Geometry: final body of the model. Coordinates: model frame, mm. A direction names the side the tool comes from. Give positions to 0.01 mm unless a question says otherwise; leave off trailing zeros. Write each loop counter-clockwise with the first axis right and the second up, starting at its lowest first coordinate (ties: lowest second). Pieces come first, ordered by that corner, then holes. Notation, with made-up numbers: M -29.75,18.25 L -11.75,18.25 A18 ccw -11.75,25.25 Z; hole C -11,19.25 d1. An arc over 180 degrees is marked long. Answer as a JSON object with one key per item and string values.
from build123d import *

# Parameters (mm, degrees)
SKETCH1_R           = 10.5
SKETCH1_R_2         = 6
BOSS_EXTRUDE1_DEPTH = 30
SKETCH2_W           = 32
SKETCH2_H           = 32
SKETCH2_R           = 6
BOSS_EXTRUDE2_DEPTH = 6
SKETCH3_R           = 2.15
CUT_EXTRUDE1_DEPTH  = 38.576588456
CHAMFER1_SIZE       = 4


with BuildPart() as part:
    # Sketch1 → Boss-Extrude1 (new body)
    with BuildSketch(Plane(origin=(0, 0, 0), x_dir=(1, 0, 0), z_dir=(0, 1, 0))):
        with Locations(Location((0, 0, 0), (0, 0, 270))):
            Circle(SKETCH1_R)
        with Locations(Location((0, 0, 0), (0, 0, 270))):
            Circle(SKETCH1_R_2, mode=Mode.SUBTRACT)
    extrude(amount=BOSS_EXTRUDE1_DEPTH)

    # Sketch2 → Boss-Extrude2 (add)
    with BuildSketch(Plane(origin=(0, 0, 0), x_dir=(1, 0, 0), z_dir=(0, 1, 0))):
        Rectangle(SKETCH2_W, SKETCH2_H)
        with Locations(Location((0, 0, 0), (0, 0, 270))):
            Circle(SKETCH2_R, mode=Mode.SUBTRACT)
    extrude(amount=BOSS_EXTRUDE2_DEPTH)

    # Sketch3 → Cut-Extrude1 (cut, through all)
    with BuildSketch(Plane(origin=(0, 0, 0), x_dir=(1, 0, 0), z_dir=(0, 1, 0))):
        with Locations(Location((-11.313708499, 11.313708499, 0), (0, 0, 270))):
            Circle(SKETCH3_R)
        with Locations(Location((-11.313708499, -11.313708499, 0), (0, 0, 270))):
            Circle(SKETCH3_R)
        with Locations(Location((11.313708499, -11.313708499, 0), (0, 0, 270))):
            Circle(SKETCH3_R)
        with Locations(Location((11.313708499, 11.313708499, 0), (0, 0, 270))):
            Circle(SKETCH3_R)
    extrude(amount=CUT_EXTRUDE1_DEPTH, mode=Mode.SUBTRACT)

    # Chamfer1
    chamfer1_edges = [part.edges().sort_by_distance(p)[0] for p in [
        (16, 3, 16),
        (16, 3, -16),
        (-16, 3, -16),
        (-16, 3, 16),
    ]]
    chamfer(chamfer1_edges, length=CHAMFER1_SIZE)


solid = part.part
1) Line query: line 1 (Y direction, x = -13, z = -9.5); line 2 (X direction, y = 10.5, z = 1); line 3 (X direction, y = 3, z = -10.5). Output: solid intervals per line, ascending. Write a range as from..to.
Geometry check:
{"line 1": "y = 0..6", "line 2": "x = -10.45..-5.92, 5.92..10.45", "line 3": "x = -16..-13.3, -9.32..9.32, 13.3..16"}
2) Pull-direction query (Z, two-part tool) for faces 1 (the flat face through (-16, 3, 0)), 2 (the flat face through (-14, 3, -14)), 3 (the cylindrical face through (12.767, 2.958, -12.898)), 4 (the flat face through (-14, 3, 14)); classes: pulls with the +Z half, pulls with the -Z half, needs draft (parallel to the pull), parting line crosses it, or undercut.
Geometry check:
{"face 1": "needs draft", "face 2": "pulls with the -Z half", "face 3": "undercut", "face 4": "pulls with the +Z half"}
3) Cut plane A-A on z = 0. Return loops of the section in (x, y), and give its area (3 significant figures).
Geometry check:
{"outline": "M -16,0 L -6,0 L -6,30 L -10.5,30 L -10.5,6 L -16,6 Z; M 6,0 L 16,0 L 16,6 L 10.5,6 L 10.5,30 L 6,30 Z", "area": "336 mm2"}
4) Set-up query: faces 5 (the cylindrical face through (3.2, 17.8, 10)), 6 (the cylindrical face through (-11.22, 2.96, -13.46)). Return all of +Z, -Z, +X, -X, +Y, -Y with unobstructed straight access to the full face (end or side cutting, diameter ignored); none if empty.
Geometry check:
{"face 5": "+Y", "face 6": "+Y, -Y"}
5) Cut plane D-D on y = 23.5. Return loops of the section in (x, z).
Geometry check:
{"outline": "C 0,0 d21; hole C 0,0 d12"}
6) Cut plane B-B on x = 0. Return loops of the section in (y, z).
Geometry check:
{"outline": "M 0,-16 L 6,-16 L 6,-10.5 L 30,-10.5 L 30,-6 L 0,-6 Z; M 0,6 L 30,6 L 30,10.5 L 6,10.5 L 6,16 L 0,16 Z"}
7) Contact query for flat-ended pins moving along their axis: P1, Ø6, axis at x = 2.5, y = 16, coming from the +Z side; P2, Ø8, axis at y = 25, z = -3.5, coming from the -X side; P3, Ø1.5, axis at x = -7.5, y = 12.5, coming from the -Z side. Output: stop coordinate, or through.
Geometry check:
{"P1": "stops at z = 10.5", "P2": "stops at x = -10.5", "P3": "stops at z = -8.04"}
8) Cut plane C-C on x = 12.5. Return loops of the section in (y, z), and give its area (3 significant figures).
Geometry check:
{"outline": "M 0,-15.5 L 6,-15.5 L 6,-13.11 L 0,-13.11 Z; M 0,-9.52 L 6,-9.52 L 6,9.52 L 0,9.52 Z; M 0,13.11 L 6,13.11 L 6,15.5 L 0,15.5 Z", "area": "143 mm2"}
